Part model, mm, in its own coordinate system. Coordinates: 2 decimals unless noted, no trailing zeros. Loops run counter-clockwise (first coordinate to the right, second up) from the corner with the lowest first, then second, coordinate; pieces in that order, holes last. Notation, with made-up numbers: (36.5, 52.25) - (84.5, 52.25) arc R5 ccw to (84.5, 57.25) - close; hole circle Ø8 at (-20.75, 58.5). An arc over 180 degrees is marked (long way). Use a Markdown table: item, result. Add a question column.
1. Band-saw the part on A-A, the plane y = 79. Give the cut face in (x, z), plus the area to 3 significant figures.
2. Band-saw the part on B-B, the plane x = -23. Give the cut face in (y, z), plus the area to 3 significant figures.
3. Band-saw the part on C-C, the plane z = 0.5. Count the separate pieces of the cut face and the enclosed holes in it, plus the area to 3 significant figures.
4. Band-saw the part on D-D, the plane x = -3.5. Give the cut face in (y, z), plus the area to 3 significant figures.
5. Drop a flat-ended pin along its axis: pin 1 (2 mm diameter, centred on x = -15, y = 79, fed in from -Z). Give the stop position or say it passes through.
6. Wall check: probe 1 along Y at (x, z) = (-18, 0.8); probe 2 along X at (y, z) = (79, 2.4); probe 3 along Y at (x, z) = (-23, 0.7). Give the ranges that are in metal, low to high. Write a range as [from, to].
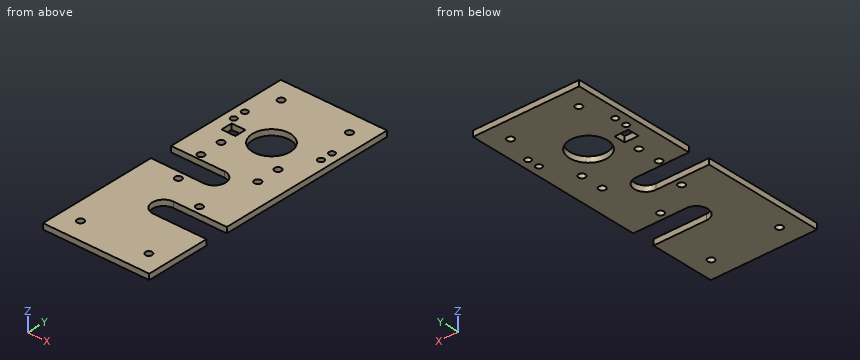
from build123d import *

# Parameters (mm, degrees)
SKETCH_R   = 10
SKETCH_R_2 = 1.8
SKETCH_R_3 = 1.6
SKETCH_W   = 7.288706
SKETCH_H   = 5.97866
PAD_DEPTH  = 3


with BuildPart() as part:
    # Sketch → Pad (new body)
    with BuildSketch(Plane.XY):
        with BuildLine():
            Line((-28, 141), (28, 141))
            Line((28, 141), (28, 46))
            Line((0, 46), (28, 46))
            ThreePointArc((0, 46), (-6, 40), (0, 34))
            Line((28, 34), (0, 34))
            Line((28, 34), (28, 0))
            Line((28, 0), (-28, 0))
            Line((-28, 0), (-28, 64))
            Line((0, 64), (-28, 64))
            ThreePointArc((0, 64), (6, 70), (0, 76))
            Line((-28, 76), (0, 76))
            Line((-28, 76), (-28, 141))
        make_face()
        with Locations((0, 104)):
            Circle(SKETCH_R, mode=Mode.SUBTRACT)
        with Locations((-18, 130)):
            Circle(SKETCH_R_2, mode=Mode.SUBTRACT)
        with Locations((18, 130)):
            Circle(SKETCH_R_2, mode=Mode.SUBTRACT)
        with Locations((-18, 11)):
            Circle(SKETCH_R_2, mode=Mode.SUBTRACT)
        with Locations((18, 11)):
            Circle(SKETCH_R_2, mode=Mode.SUBTRACT)
        with Locations((-23, 114)):
            Circle(SKETCH_R_3, mode=Mode.SUBTRACT)
        with Locations((-23, 107.5)):
            Circle(SKETCH_R_3, mode=Mode.SUBTRACT)
        with Locations((23, 114)):
            Circle(SKETCH_R_3, mode=Mode.SUBTRACT)
        with Locations((23, 107.5)):
            Circle(SKETCH_R_3, mode=Mode.SUBTRACT)
        with Locations((-10, 60)):
            Circle(SKETCH_R_2, mode=Mode.SUBTRACT)
        with Locations((10, 50)):
            Circle(SKETCH_R_2, mode=Mode.SUBTRACT)
        with Locations((-15, 91)):
            Circle(SKETCH_R_2, mode=Mode.SUBTRACT)
        with Locations((-15, 79)):
            Circle(SKETCH_R_2, mode=Mode.SUBTRACT)
        with Locations((15, 91)):
            Circle(SKETCH_R_2, mode=Mode.SUBTRACT)
        with Locations((15, 79)):
            Circle(SKETCH_R_2, mode=Mode.SUBTRACT)
        with Locations((-17.587784, 101.235753)):
            Rectangle(SKETCH_W, SKETCH_H, mode=Mode.SUBTRACT)
    extrude(amount=PAD_DEPTH)


solid = part.part
Geometry check:
| question | item | result |
|---|---|---|
| 1 | outline | (-28, 0) - (-16.8, 0) - (-16.8, 3) - (-28, 3) - close; (-13.2, 0) - (13.2, 0) - (13.2, 3) - (-13.2, 3) - close; (16.8, 0) - (28, 0) - (28, 3) - (16.8, 3) - close |
| 1 | area | 146 mm^2 |
| 2 | outline | (0, 0) - (64, 0) - (64, 3) - (0, 3) - close; (76, 0) - (105.9, 0) - (105.9, 3) - (76, 3) - close; (109.1, 0) - (112.4, 0) - (112.4, 3) - (109.1, 3) - close; (115.6, 0) - (141, 0) - (141, 3) - (115.6, 3) - close |
| 2 | area | 368 mm^2 |
| 3 | separate pieces | 1 |
| 3 | enclosed holes | 16 |
| 3 | area | 6,620 mm^2 |
| 4 | outline | (0, 0) - (35.13, 0) - (35.13, 3) - (0, 3) - close; (44.87, 0) - (64, 0) - (64, 3) - (44.87, 3) - close; (76, 0) - (94.63, 0) - (94.63, 3) - (76, 3) - close; (113.37, 0) - (141, 0) - (141, 3) - (113.37, 3) - close |
| 4 | area | 302 mm^2 |
| 5 | pin 1 | passes through |
| 6 | probe 1 | y = [0, 9.2], [12.8, 64], [76, 98.25], [104.23, 128.2], [131.8, 141] |
| 6 | probe 2 | x = [-28, -16.8], [-13.2, 13.2], [16.8, 28] |
| 6 | probe 3 | y = [0, 64], [76, 105.9], [109.1, 112.4], [115.6, 141] |
